```python
from build123d import *

# Parameters (mm, degrees)
SKETCH_1_R          = 1.5
EXTRUDE_1_DEPTH     = 12
SKETCH_2_R          = 3
EXTRUDE_2_DEPTH     = 3
CHAMFER_1_SIZE      = 2.9
CUT_EXTRUDE_1_DEPTH = 1


with BuildPart() as part:
    # 草图1 → 凸台-拉伸1 (new body)
    with BuildSketch(Plane(origin=(0, 0, 0), x_dir=(1, 0, 0), z_dir=(0, 1, 0))):
        with Locations(Location((0, 0, 0), (0, 0, 270))):
            Circle(SKETCH_1_R)
    extrude(amount=EXTRUDE_1_DEPTH)

    # 草图2 → 凸台-拉伸2 (add)
    with BuildSketch(Plane(origin=(0, 12, 0), x_dir=(1, 0, 0), z_dir=(0, 1, 0))):
        with Locations(Location((0, 0, 0), (0, 0, 270))):
            Circle(SKETCH_2_R)
    extrude(amount=EXTRUDE_2_DEPTH)

    # 倒角1
    # the kernel refuses this chamfer: 2.9 mm, written as the material it takes off along each edge
    with BuildSketch(Plane(origin=(0, 12, 0), x_dir=(0, 0, 1), z_dir=(-1, 0, 0))) as chamfer_1_piece_1_section:
        Polygon((3, CHAMFER_1_SIZE), (3 - CHAMFER_1_SIZE, 0), (3, 0), align=None)
    chamfer_1_piece_1 = revolve(axis=Axis((0, 12, 0), (0, 1, 0)), mode=Mode.PRIVATE)
    chamfer_1_piece_1 = chamfer_1_piece_1 - Plane(origin=(0, 14.16453564, 0), x_dir=(0, 0, 1), z_dir=(0, -1, 0)) * Cylinder(1.5, 12, mode=Mode.PRIVATE)
    add(chamfer_1_piece_1, mode=Mode.SUBTRACT)

    # 草图3 → 切除-拉伸1 (cut)
    with BuildSketch(Plane(origin=(0, 15, 0), x_dir=(1, 0, 0), z_dir=(0, 1, 0))):
        Polygon((1.017530084, -0.545862493), (0.981495828, 0.608275655), (-0.036034256, 1.154138148), (-1.017530084, 0.545862493), (-0.981495828, -0.608275655), (0.036034256, -1.154138148), align=None)
    extrude(amount=-CUT_EXTRUDE_1_DEPTH, mode=Mode.SUBTRACT)


solid = part.part
```
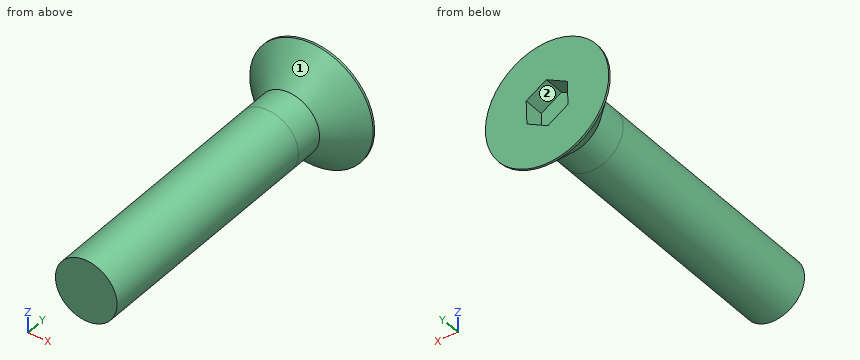
Build history of the part. All positions in model axes, mm. Face numbers are marked on the shaded views. A direction names the side the tool comes from. Give positions to 0.01 mm unless a question says otherwise; leave off trailing zeros. Loops run counter-clockwise (first coordinate to the right, second up) from the corner with the lowest first, then second, coordinate; pieces in that order, holes last.
Item 1: Flat gauge pin, fed straight in: pin 1 (2 mm diameter, centred on y = 3.5, z = 0.5, fed in from +X). Where does the tip first touch, or does it go through?
Answers follow:
pin 1: stops at x = 1.5
Item 2: Which spindle directions (+Z, -Z, +X, -X, +Y, -Y) get a long thin tool onto all of the face, cutting with end or side? Do the marked faces 1 and 2. Say none if no direction does.
Answers follow:
face 1: -Y
face 2: +Y
Item 3: Slice it at A-A, the plane z = 0. List the corners of the cut face in (x, y), and give its area (3 significant figures).
Answers follow:
outline: (-3, 14.9) - (-1.5, 13.4) - (-1.5, 0) - (1.5, 0) - (1.5, 13.4) - (3, 14.9) - (3, 15) - (1, 15) - (1, 14) - (-1, 14) - (-1, 15) - (-3, 15) - close
area: 45.5 mm2
Item 4: Drill centre lines: line 1 (X direction, y = 3.75, z = -1.1); line 2 (Y direction, x = 1.5, z = -2). Where is each one in solid material? Low to high.
Answers follow:
line 1: x = -1.02 to 1.02
line 2: y = 14.4 to 15
Item 5: Slice it at B-B, the plane y = 3.75. List the corners of the cut face in (x, z).
Answers follow:
outline: circle Ø3 at (0, 0)
